Part model, mm, in its own coordinate system. Face numbers are marked on the shaded views. A direction names the side the tool comes from. Give positions to 0.01 mm unless a question says otherwise; leave off trailing zeros. Order: outer loops, then holes, each group sorted by start corner. A loop starts at its lowest first (then second) coordinate and runs counter-clockwise, first axis right, second up. Notation, with made-up numbers: (75, 22) - (93, 22) arc R21 cw to (93, 49) - close; hole circle Ø9 at (51, 50). An arc over 180 degrees is marked (long way). Use a Markdown table: item, result. Add a question column.
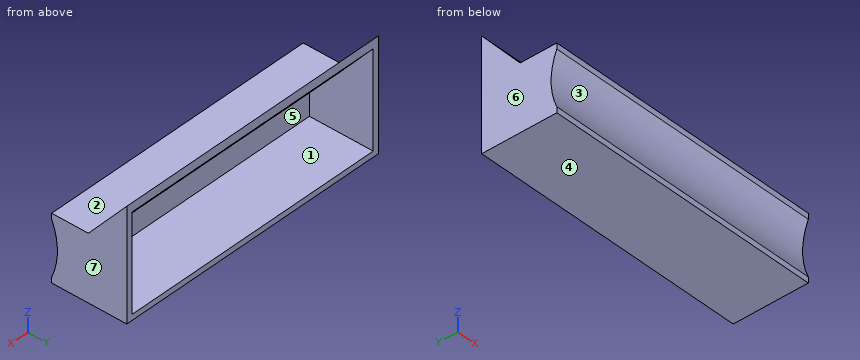
Autodesk Inventor part; units mm, degrees
ref_plane "YZ Plane" through (0, 0, 0) normal (1, 0, 0) x (0, 1, 0)
ref_plane "XZ Plane" through (0, 0, 0) normal (0, 1, 0) x (-1, 0, 0)
ref_plane "XY Plane" through (0, 0, 0) normal (0, 0, 1) x (1, 0, 0)
ref_plane "Work Plane1" through (0, 0, 0) normal (0, 0, 1) x (1, 0, 0)
ref_plane "Work Plane2" through (157.5, -135.5375, 119.9) normal (1, 0, 0) x (0, 0, -1)
ref_plane "Work Plane3" through (404.675, -135.5375, 119.9) normal (-1, 0, 0) x (0, 0, 1)
sketch "Sketch2" plane through (404.675, -135.5375, 119.9) normal (-1, 0, 0) x (0, 0, 1)
  line L0 (-120, -33.125) -> (-120, 33.125)
  line L1 (120, -33.125) -> (-120, -33.125)
  line L2 (120, 33.125) -> (120, -33.125)
  line L3 (-120, 33.125) -> (120, 33.125)
  circle A0 centre (7, 26.125) radius 1.95
  circle A1 centre (113, -26.875) radius 1.95
  circle A2 centre (113, 12.125) radius 1.95
  circle A3 centre (99, 26.125) radius 1.95
  circle A4 centre (-55, -26.875) radius 1.95
  line L4 (0.75, 33.125) -> (-62, -20.125)
  line L5 (-50.0649, 0.1287) -> (-21.3323, 24.6904)
  line L6 (-11.7313, 32.1577) -> (-59.0108, -8.2587)
  line L7 (-62, -22.3139) -> (-62, -29.97)
  line L8 (-119.9, -33.125) -> (-62.2, -33.125)
  line L9 (-62.2, -33.125) -> (-62.2, 33.125)
  line L10 (-62.2, 33.125) -> (-119.9, 33.125)
  line L11 (-119.9, 33.125) -> (-119.9, -33.125)
  line L12 (-62.2, 33.125) -> (-22.5461, 33.125)
  line L13 (-22.5461, 33.125) -> (-62.2, -0.7727)
  line L14 (-50.1997, 8.8278) -> (-29.9045, 26.1769)
  point P0 (-119.9, 135.5375)
  point P1 (-119.9, 33.125)
  point P2 (-119.9, -33.125)
  point P3 (-62.2, -33.125)
  dimension "d2" = 0.1
  dimension "d3" = 0.2
  dimension "d16" = 0.5
extrude "Extrusion1" add sketch "Sketch2" along normal up to surface (247.175 mm away) contours L11 L3 L9 L1 | L3 L13 L9
shell "Shell1" thickness 5 removed faces 1 at (322.2833, -102.4125, 64.9026)
sketch "Sketch3" plane through (404.675, -135.5375, 119.9) normal (1, 0, 0) x (0, 0, -1)
  line L0 (114.9, -28.125) -> (67.2, -28.125)
  line L1 (67.2, -28.125) -> (67.2, 1.531)
  line L2 (115, 28.125) -> (115, -28.125)
  line L3 (67.2, -23.125) -> (115, -23.125)
  line L4 (115, -23.125) -> (115, -28.125)
  line L5 (115, -28.125) -> (67.2, -28.125)
  line L6 (67.2, -28.125) -> (67.2, -23.125)
  point P0 (119.9, 135.5375)
  point P1 (115, -23.125)
  dimension "d8" = 5
extrude "Extrusion2" add sketch "Sketch3" against normal up to surface (242.175 mm away)
sketch "Sketch4" plane through (404.675, -135.5375, 119.9) normal (1, 0, 0) x (0, 0, -1)
  line L0 (119.9, -33.125) -> (62.2, -33.125)
  arc A0 (114.9, -33.125) -> (67.2, -33.125) centre (91.05, -87.5073) ccw
  point P0 (119.9, 135.5375)
  point P1 (91.05, -28.125)
  point P2 (91.05, -33.125)
  dimension "d12" = 5
  dimension "d13" = 5
extrude "Extrusion3" cut sketch "Sketch4" against normal through all
properties part number "sump"
1. Cut at A-A (y = -151). Write the cut outline in (x, z) (3 decimals), plus the area to 3 significant figures.
2. Cut at C-C (z = 45). Write the cut outline in (x, y) (1 decimal), plus the area to 3 significant figures.
3. Cut at D-D (y = -121). Write the cut outline in (x, z) (3 decimals), plus the area to 3 significant figures.
4. Cut at B-B (x = 330.5). Write the cut outline in (y, z).
5. Drill centre lines: probe 1 along X at (y, z) = (-109, 31.5) (3 decimals); probe 2 along Z at (x, y) = (382.5, -148); probe 3 along Z at (x, y) = (178, -136). Where is each one in solid material? Low to high. Write a range as [from, to].
6. Mould opens along X. For the marked faces 4, 5, 6 and 7 say: released by +X, released by -X, zero draft, split by the parting line, or undercut.
7. Tool access for the marked faces 1, 2 and 3: list every direction of +Z, -Z, +X, -X, +Y, -Y with a clear straight run to the whole face (end or side of a thin tool).
8. Pin check, flat tips, straight feed: P1, Ø10, axis at y = -157, z = 64.5, coming from the +X side; P2, Ø10, axis at x = 325, z = 19.5, coming from the +Y side; P3, Ø2, axis at x = 215.5, y = -129, coming from the +Z side; P4, Ø2, axis at x = 229, z = 83, coming from the -Y side. Stop position of each tip, or through.
Responses:
| question | item | result |
|---|---|---|
| 1 | outline | (157.5, 0) - (404.675, 0) - (404.675, 57.7) - (157.5, 57.7) - close; hole (162.5, 5) - (399.675, 5) - (399.675, 52.7) - (162.5, 52.7) - close |
| 1 | area | 2,950 mm² |
| 2 | outline | (157.5, -165.9) - (404.7, -165.9) - (404.7, -102.4) - (399.7, -102.4) - (399.7, -158.7) - (162.5, -158.7) - (162.5, -102.4) - (157.5, -102.4) - close |
| 2 | area | 2,350 mm² |
| 3 | outline | (157.5, 0) - (404.675, 0) - (404.675, 75.61) - (157.5, 75.61) - close; hole (162.5, 5) - (399.675, 5) - (399.675, 67.915) - (162.5, 67.915) - close |
| 3 | area | 3,770 mm² |
| 4 | outline | (-168.66, 0) - (-102.41, 0) - (-102.41, 5) - (-158.66, 5) - (-158.66, 52.7) - (-134.01, 52.7) - (-102.41, 89.66) - (-102.41, 97.35) - (-136.31, 57.7) - (-168.66, 57.7) - (-168.66, 52.7) arc R59.38 cw to (-168.66, 5) - close |
| 5 | probe 1 | x = [157.5, 162.5], [399.675, 404.675] |
| 5 | probe 2 | z = [0, 5], [52.7, 57.7] |
| 5 | probe 3 | z = [0, 5], [52.7, 58.06] |
| 6 | face 4 | zero draft |
| 6 | face 5 | undercut |
| 6 | face 6 | released by -X |
| 6 | face 7 | released by +X |
| 7 | face 1 | +Y |
| 7 | face 2 | +Z, +X, -X, -Y |
| 7 | face 3 | +X, -X, -Y |
| 8 | P1 | passes through |
| 8 | P2 | stops at y = -158.66 |
| 8 | P3 | stops at z = 67.42 |
| 8 | P4 | stops at y = -115.54 |
